from build123d import *

# Parameters (mm, degrees)
SKETCH1_W           = 50
SKETCH1_H           = 50
SKETCH1_R           = 2.81
BOSS_EXTRUDE1_DEPTH = 1
SKETCH2_W           = 50
SKETCH2_H           = 50
BOSS_EXTRUDE2_DEPTH = 3


with BuildPart() as part:
    # Sketch1 → Boss-Extrude1 (new body)
    with BuildSketch(Plane.XY):
        with Locations((15, -15)):
            Rectangle(SKETCH1_W, SKETCH1_H)
        Circle(SKETCH1_R, mode=Mode.SUBTRACT)
        with Locations((10, 0)):
            Circle(SKETCH1_R, mode=Mode.SUBTRACT)
        with Locations((20, 0)):
            Circle(SKETCH1_R, mode=Mode.SUBTRACT)
        with Locations((30, 0)):
            Circle(SKETCH1_R, mode=Mode.SUBTRACT)
        with Locations((10, -10)):
            Circle(SKETCH1_R, mode=Mode.SUBTRACT)
        with Locations((20, -10)):
            Circle(SKETCH1_R, mode=Mode.SUBTRACT)
        with Locations((30, -10)):
            Circle(SKETCH1_R, mode=Mode.SUBTRACT)
        with Locations((10, -20)):
            Circle(SKETCH1_R, mode=Mode.SUBTRACT)
        with Locations((20, -20)):
            Circle(SKETCH1_R, mode=Mode.SUBTRACT)
        with Locations((30, -20)):
            Circle(SKETCH1_R, mode=Mode.SUBTRACT)
        with Locations((10, -30)):
            Circle(SKETCH1_R, mode=Mode.SUBTRACT)
        with Locations((20, -30)):
            Circle(SKETCH1_R, mode=Mode.SUBTRACT)
        with Locations((30, -30)):
            Circle(SKETCH1_R, mode=Mode.SUBTRACT)
        with Locations((0, -10)):
            Circle(SKETCH1_R, mode=Mode.SUBTRACT)
        with Locations((0, -20)):
            Circle(SKETCH1_R, mode=Mode.SUBTRACT)
        with Locations((0, -30)):
            Circle(SKETCH1_R, mode=Mode.SUBTRACT)
    extrude(amount=BOSS_EXTRUDE1_DEPTH)

    # Sketch2 → Boss-Extrude2 (add)
    with BuildSketch(Plane(origin=(0, 0, 0), x_dir=(-1, 0, 0), z_dir=(0, 0, -1))):
        with Locations((-15, -15)):
            Rectangle(SKETCH2_W, SKETCH2_H)
    extrude(amount=BOSS_EXTRUDE2_DEPTH)


solid = part.part
Model file for the job. Use its own axes, mm. A direction names the side the tool comes from. Give positions to 0.01 mm unless a question says otherwise; leave off trailing zeros. Order: outer loops, then holes, each group sorted by start corner. A loop starts at its lowest first (then second) coordinate and runs counter-clockwise, first axis right, second up. Notation, with made-up numbers: (8.25, 33.25) - (27.25, 33.25) arc R16 cw to (27.25, 38.25) - close; hole circle Ø9 at (38.5, 85). An arc over 180 degrees is marked (long way). One line per item, written item: value.
Item 1: Two-plate mould, pull along X, no slides. Class faces 1 (the flat face through (40, -15, -1)), 2 (the flat face through (15, -15, -3)), 3 (the flat face through (10, -20, 0)): released by +X, released by -X, zero draft, split by the parting line, or undercut.
Response values:
face 1: released by +X
face 2: zero draft
face 3: undercut
Item 2: Pin check, flat tips, straight feed: pin 1 Ø3 at (x, y) = (29, -28.5) entering from +Z; pin 2 Ø4.5 at (x, y) = (20, -19.5) entering from +Z. Stop position of each tip, or through.
Response values:
pin 1: z = 1
pin 2: z = 0
Item 3: Wall check: line 1 (Y direction, x = 10, z = 0.5); line 2 (X direction, y = -28, z = 0.2); line 3 (Z direction, x = 31, y = -0.5). Give the ranges that are in metal, low to high.
Response values:
line 1: -40 to -32.81, -27.19 to -22.81, -17.19 to -12.81, -7.19 to -2.81, 2.81 to 10
line 2: -10 to -1.97, 1.97 to 8.03, 11.97 to 18.03, 21.97 to 28.03, 31.97 to 40
line 3: -3 to 0
Item 4: Slice it at B-B (x = 20). List the corners of the cut face in (y, z), then the cut area to 3 significant figures.
Response values:
outline: (-40, -3) - (10, -3) - (10, 1) - (2.81, 1) - (2.81, 0) - (-2.81, 0) - (-2.81, 1) - (-7.19, 1) - (-7.19, 0) - (-12.81, 0) - (-12.81, 1) - (-17.19, 1) - (-17.19, 0) - (-22.81, 0) - (-22.81, 1) - (-27.19, 1) - (-27.19, 0) - (-32.81, 0) - (-32.81, 1) - (-40, 1) - close
area: 178 mm2
Item 5: Slice it at A-A (y = -20). List the corners of the cut face in (x, z), then the cut area to 3 significant figures.
Response values:
outline: (-10, -3) - (40, -3) - (40, 1) - (32.81, 1) - (32.81, 0) - (27.19, 0) - (27.19, 1) - (22.81, 1) - (22.81, 0) - (17.19, 0) - (17.19, 1) - (12.81, 1) - (12.81, 0) - (7.19, 0) - (7.19, 1) - (2.81, 1) - (2.81, 0) - (-2.81, 0) - (-2.81, 1) - (-10, 1) - close
area: 178 mm2
Item 6: Tool access for faces 4 (the cylindrical face through (27.193, 0.124, 0.493)), 5 (the flat face through (15, -40, -1)): list every direction of +Z, -Z, +X, -X, +Y, -Y with a clear straight run to the whole face (end or side of a thin tool).
Response values:
face 4: +Z
face 5: +Z, -Z, +X, -X, -Y
